Geometry: final body of the model. Coordinates: model frame, mm. A direction names the side the tool comes from. Round coordinates to 2 decimals unless told otherwise and drop trailing zeros. Loops run counter-clockwise (first coordinate to the right, second up) from the corner with the lowest first, then second, coordinate; pieces in that order, holes last. Notation, with made-up numbers: (-36, 5) - (14, 5) arc R25 ccw to (14, 24) - close; hole circle Ø2 at (70, 49). An arc over 180 degrees is marked (long way). Use CSV: the item, a comma, the result in double quotes.
from build123d import *

# Parameters (mm, degrees)
SKETCH2_W           = 142
SKETCH2_H           = 46
SKETCH2_R           = 1.6
BOSS_EXTRUDE1_DEPTH = 3
SKETCH3_R           = 1.6
CUT_EXTRUDE1_DEPTH  = 4
SKETCH3_3_R         = 1.6
SKETCH3_3_W         = 11
SKETCH3_3_H         = 9
BOSS_EXTRUDE2_DEPTH = 3
FILLET2_R           = 2
FILLET3_R           = 2
FILLET4_R           = 10


with BuildPart() as part:
    # Sketch2 → Boss-Extrude1 (new body)
    with BuildSketch(Plane.XY):
        with Locations((15, 0)):
            Rectangle(SKETCH2_W, SKETCH2_H)
        with Locations((-25, -14)):
            Circle(SKETCH2_R, mode=Mode.SUBTRACT)
        with Locations((45, -14)):
            Circle(SKETCH2_R, mode=Mode.SUBTRACT)
        with Locations((-25, 14)):
            Circle(SKETCH2_R, mode=Mode.SUBTRACT)
        with Locations((45, 14)):
            Circle(SKETCH2_R, mode=Mode.SUBTRACT)
    extrude(amount=BOSS_EXTRUDE1_DEPTH)

    # Sketch3 → Cut-Extrude1 (cut, through all)
    with BuildSketch(Plane.XY.offset(3)):
        with BuildLine():
            Line((86, -14), (86, 14))
            ThreePointArc((86, 14), (72, 0), (86, -14))
        make_face()
        with Locations((82, 19)):
            Circle(SKETCH3_R)
        with Locations((56, 19)):
            Circle(SKETCH3_R)
        with Locations((-44, 19)):
            Circle(SKETCH3_R)
        with Locations((70, 19)):
            Circle(SKETCH3_R)
        with Locations((82, -19)):
            Circle(SKETCH3_R)
        with Locations((70, -19)):
            Circle(SKETCH3_R)
        with Locations((-44, -19)):
            Circle(SKETCH3_R)
        with Locations((56, -19)):
            Circle(SKETCH3_R)
    extrude(amount=-CUT_EXTRUDE1_DEPTH, mode=Mode.SUBTRACT)

    # Sketch3<3> → Boss-Extrude2 (add)
    with BuildSketch(Plane.XY.offset(3)):
        Polygon((97, 23), (86, 23), (86, 19), (86, 14), (97, 14), align=None)
        with Locations((94, 19)):
            Circle(SKETCH3_3_R, mode=Mode.SUBTRACT)
        with Locations((91.5, -18.5)):
            Rectangle(SKETCH3_3_W, SKETCH3_3_H)
        with Locations((94, -19)):
            Circle(SKETCH3_3_R, mode=Mode.SUBTRACT)
    extrude(amount=-BOSS_EXTRUDE2_DEPTH)

    # Fillet2
    fillet2_edges = [part.edges().sort_by_distance(p)[0] for p in [
        (97, 23, 1.5),
        (97, -23, 1.5),
    ]]
    fillet(fillet2_edges, radius=FILLET2_R)

    # Fillet3
    fillet3_edges = [part.edges().sort_by_distance(p)[0] for p in [
        (97, 14, 1.5),
        (97, -14, 1.5),
    ]]
    fillet(fillet3_edges, radius=FILLET3_R)

    # Fillet4
    fillet4_edges = [part.edges().sort_by_distance(p)[0] for p in [
        (-56, 23, 1.5),
        (-56, -23, 1.5),
    ]]
    fillet(fillet4_edges, radius=FILLET4_R)


solid = part.part
Item 1: Pin query (flat end, axial travel): P1, Ø1, axis at y = -9, z = 2, coming from the +X side. Return the tip coordinate at first contact, or that it passes through.
Final values:
P1,"stops at x = 75.72"
Item 2: Material intervals for line 1 (Y direction, x = 56, z = 1.7); line 2 (Y direction, x = 45, z = 1.4); line 3 (Y direction, x = 94, z = 1.15), sorted ascending.
Final values:
line 1,"y = -23 to -20.6, -17.4 to 17.4, 20.6 to 23"
line 2,"y = -23 to -15.6, -12.4 to 12.4, 15.6 to 23"
line 3,"y = -23 to -20.6, -17.4 to -14, 14 to 17.4, 20.6 to 23"
Item 3: Section C-C on z = 0.45. Give the number of separate pieces and of enclosed holes in the cut face, plus the area to 3 significant figures.
Final values:
separate pieces,"1"
enclosed holes,"14"
area,"6,260 mm²"
Item 4: Section A-A on y = 19. Return the cut outline in (x, z), plus the area to 3 significant figures.
Final values:
outline,"(-54, 0) - (-45.6, 0) - (-45.6, 3) - (-54, 3) - close; (-42.4, 0) - (54.4, 0) - (54.4, 3) - (-42.4, 3) - close; (57.6, 0) - (68.4, 0) - (68.4, 3) - (57.6, 3) - close; (71.6, 0) - (80.4, 0) - (80.4, 3) - (71.6, 3) - close; (83.6, 0) - (92.4, 0) - (92.4, 3) - (83.6, 3) - close; (95.6, 0) - (97, 0) - (97, 3) - (95.6, 3) - close"
area,"405 mm²"
Item 5: Section D-D on y = 5. Return the cut outline in (x, z), plus the area to 3 significant figures.
Final values:
outline,"(-56, 0) - (72.92, 0) - (72.92, 3) - (-56, 3) - close"
area,"387 mm²"
Item 6: Mould query, pull axis X, two halves, no side actions, for faces 3 (the flat face through (-56, 0, 1)), 4 (the cylindrical face through (44.792, 15.586, 1.479)), 5 (the flat face through (97, 18, 2)), 6 (the flat face through (25, 23, 2)). Classes: released by +X, released by -X, zero draft, split by the parting line, or undercut.
Final values:
face 3,"released by -X"
face 4,"undercut"
face 5,"released by +X"
face 6,"zero draft"
Item 7: Reachability of faces 1 (the flat face through (90, -14, 2)), 2 (the cylindrical face through (-44.208, 20.586, 1.521)) from +Z, -Z, +X, -X, +Y, -Y: full face, straight path, thin tool, end or side. Return the list, or none.
Final values:
face 1,"+Z, -Z, +X"
face 2,"+Z, -Z"
Item 8: Section B-B on x = -25. Return the cut outline in (y, z), plus the area to 3 significant figures.
Final values:
outline,"(-23, 0) - (-15.6, 0) - (-15.6, 3) - (-23, 3) - close; (-12.4, 0) - (12.4, 0) - (12.4, 3) - (-12.4, 3) - close; (15.6, 0) - (23, 0) - (23, 3) - (15.6, 3) - close"
area,"119 mm²"
